For this review, use the dimensioned drawing (mm, ordinates from the lowest corner) and the shaded views. A direction names the side the tool comes from. Coordinates: 2 decimals unless noted, no trailing zeros. Loops run counter-clockwise (first coordinate to the right, second up) from the corner with the lowest first, then second, coordinate; pieces in that order, holes last. Notation, with made-up numbers: (88, 6) - (139, 6) arc R33 cw to (139, 37) - close; hole circle Ø9 at (-2, 36). An arc over 180 degrees is marked (long way). Answer in a Markdown table with one row per item. Add a question column.
(1) We need section A-A, the plane x = 34. Write out the cut boundary in (y, z).
(2) We need section D-D, the plane x = 46.5. Write out the cut boundary in (y, z), plus the area to 3 significant figures.
(3) We need section B-B, the plane z = 9.5. Write out the cut boundary in (x, y) (1 decimal), plus the area to 3 significant figures.
(4) Clearance check with flat-ended pins moving along their axes: pin 1 (8 mm diameter, centred on x = 27.5, y = 10.5, fed in from -Z); pin 2 (6.5 mm diameter, centred on y = 21.5, z = 6.5, fed in from +X); pin 3 (2 mm diameter, centred on x = 51, z = 8.5, fed in from +Y); pin 4 (7.5 mm diameter, centred on y = 60, z = 16.5, fed in from +X) (1 decimal). State where each tip first meets the part, or that it passes through.
(5) We need section C-C, the plane y = 32. Write out the cut boundary in (x, z) (1 decimal), plus the area to 3 significant figures.
(6) To check wall thickness, follow L1, parallel to Y at x = 35.5, z = 14; L2, parallel to X at y = 54, z = 11.5 (1 decimal); L3, parallel to Y at x = 41.5, z = 11.5 (1 decimal). State the ranges of each line that lie inside material, in increasing order. Write a range as [from, to].
(7) For the marked faces 1, 2 and 3, list the 3-axis set-ups (+Z, -Z, +X, -X, +Y, -Y) from which the entire face can be reached by the end or side of a thin tool; tool diameter is ignored.
(8) The part is to be moulded in two halves that separate along Y. For the marked faces 4, 5 and 6, say which applies: released by +Y, released by -Y, zero draft, split by the parting line, or undercut.
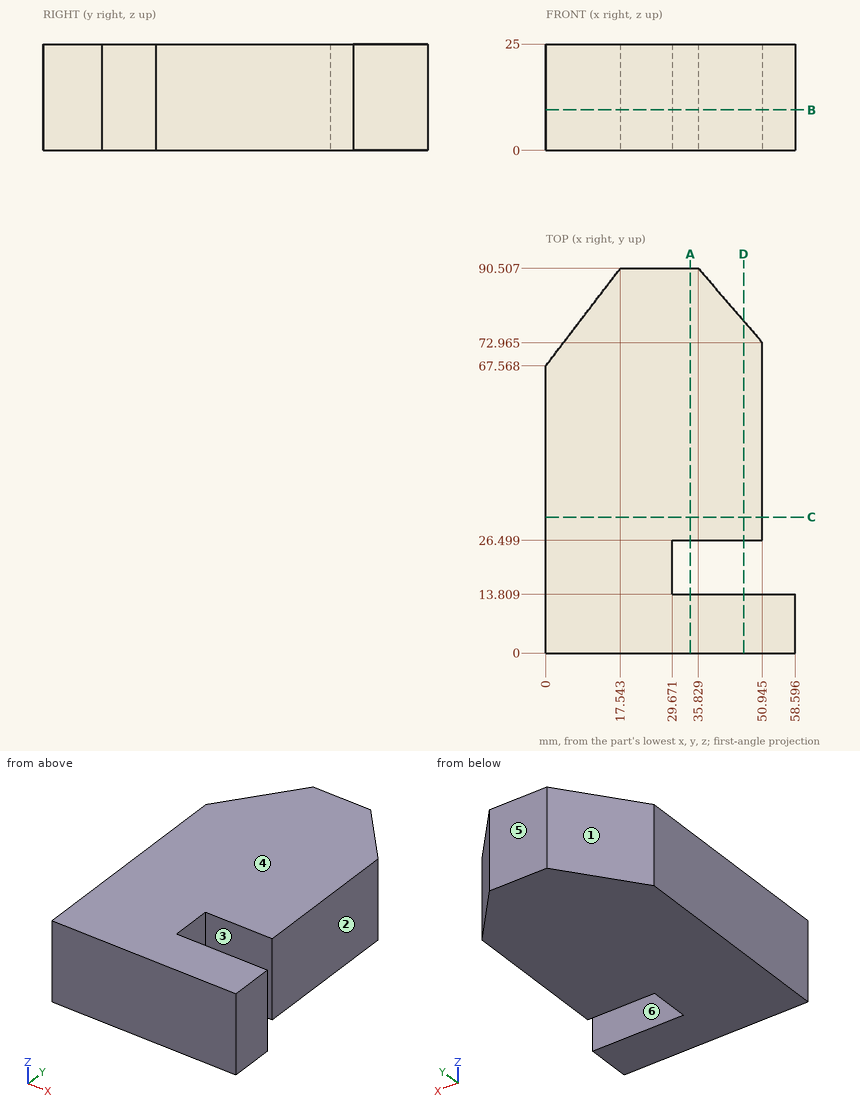
Responses:
| question | item | result |
|---|---|---|
| 1 | outline | (0, 0) - (13.81, 0) - (13.81, 25) - (0, 25) - close; (26.5, 0) - (90.51, 0) - (90.51, 25) - (26.5, 25) - close |
| 2 | outline | (0, 0) - (13.81, 0) - (13.81, 25) - (0, 25) - close; (26.5, 0) - (78.12, 0) - (78.12, 25) - (26.5, 25) - close |
| 2 | area | 1,640 mm2 |
| 3 | outline | (0, 0) - (58.6, 0) - (58.6, 13.8) - (29.7, 13.8) - (29.7, 26.5) - (50.9, 26.5) - (50.9, 73) - (35.8, 90.5) - (17.5, 90.5) - (0, 67.6) - close |
| 3 | area | 4,110 mm2 |
| 4 | pin 1 | stops at z = 0 |
| 4 | pin 2 | stops at x = 29.67 |
| 4 | pin 3 | stops at y = 74.06 |
| 4 | pin 4 | stops at x = 50.9 |
| 5 | outline | (0, 0) - (50.9, 0) - (50.9, 25) - (0, 25) - close |
| 5 | area | 1,270 mm2 |
| 6 | L1 | y = [0, 13.81], [26.5, 90.51] |
| 6 | L2 | x = [0, 50.9] |
| 6 | L3 | y = [0, 13.8], [26.5, 83.9] |
| 7 | face 1 | +Z, -Z, -X, +Y |
| 7 | face 2 | +Z, -Z, +X, +Y |
| 7 | face 3 | +Z, -Z, +X |
| 8 | face 4 | zero draft |
| 8 | face 5 | released by +Y |
| 8 | face 6 | undercut |
